Answer from the drawing. Dimensions are ordinates in mm from the lowest x, y and z of the part. Coordinates: 2 decimals unless noted, no trailing zeros. Write each loop counter-clockwise with the first axis right and the second up, starting at its lowest first coordinate (ties: lowest second). Pieces come first, ordered by that corner, then holes.
(1) Straight lines are drawn through the part: line 1 along Z through (x, y) = (624.5, 139.5); line 2 along Y through (x, z) = (208, 2.5); line 3 along Y through (x, z) = (286, 24). For each, find the intervals that lie inside material, in ascending order.
(2) The part is cut by section C-C, the plane z = 20.5. Determine the outline of the cut face in (x, y), and give its area (3 significant figures).
(3) Given pin 1 (4 mm diameter, centred on x = 1163, z = 15, fed in from +Y); pin 2 (6 mm diameter, centred on y = 124, z = 3.5, fed in from +X); pin 3 (6 mm diameter, centred on y = 107, z = 7, fed in from -X), each flat-ended and moving along its own axis, determine where each tip first touches the part or whether it passes through.
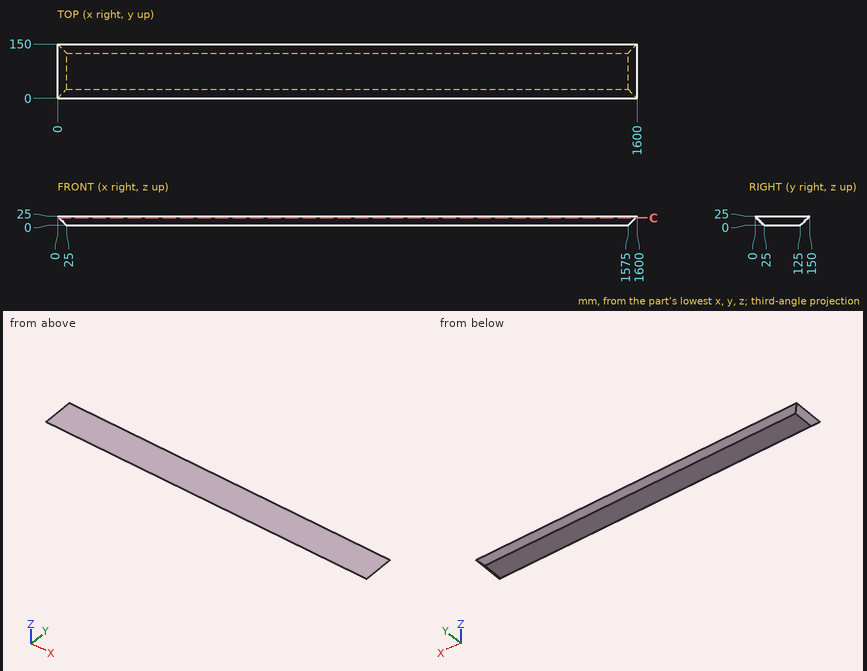
Computed:
1. line 1: z = 14.5 to 25
1. line 2: y = 22.5 to 127.5
1. line 3: y = 1 to 149
2. outline: (4.5, 4.5) - (1595.5, 4.5) - (1595.5, 145.5) - (4.5, 145.5) - close
2. area: 224,000 mm2
3. pin 1: stops at y = 142
3. pin 2: stops at x = 1581.5
3. pin 3: stops at x = 15
